Design review of the part built by this model. Coordinates are the model's own, in mm. Round coordinates to 2 decimals unless told otherwise and drop trailing zeros. Loops run counter-clockwise (first coordinate to the right, second up) from the corner with the lowest first, then second, coordinate; pieces in that order, holes last. Notation, with made-up numbers: M 79.25,12.25 L 94.25,12.25 A26 cw 94.25,51.25 Z; hole C 0,42 d8. An arc over 180 degrees is marked long. One line per item, written item: value. Start each with the question number.
Item 1: For line 1 along Z through (x, y) = (-5.5, 31.5); line 2 along Y through (x, z) = (1.75, 0); line 3 along Z through (x, y) = (5.5, -10.5), list the stretches that pass through material, from the lowest coordinate up.
Item 2: Clearance check with flat-ended pins moving along their axes: pin 1 (1.5 mm diameter, centred on x = -5, z = -13, fed in from -Y); pin 2 (6 mm diameter, centred on x = -0.5, y = 47.5, fed in from +Z); pin 3 (8 mm diameter, centred on x = -0.5, z = -27.5, fed in from +Y); pin 4 (6 mm diameter, centred on x = -4, z = -5.5, fed in from +Y). State where each tip first meets the part, or that it passes through.
Item 3: We need section C-C (z = 2.5). Write out the cut boundary in (x, y).
Item 4: We need section A-A (x = -3.25). Write out the cut boundary in (y, z), then the cut area to 3 significant figures.
Item 5: We need section B-B (y = -5). Write out the cut boundary in (x, z).
from build123d import *

# Parameters (mm, degrees)
BOSS_EXTRU_1_DEPTH      = 10
BOSS_EXTRU_1_DEPTH_BACK = 10
ESQUISSE1_R             = 1


with BuildPart() as part:
    # Esquisse1 → Boss.-Extru.1 (new, two sides: drawn at the far end of the back side and taken through both)
    with BuildSketch(Plane(origin=(0, 0, 0), x_dir=(0, 0, -1), z_dir=(1, 0, 0)).offset(-BOSS_EXTRU_1_DEPTH_BACK)):
        Polygon((5.047823589, 2.497154895), (33.133709904, -54.276495693), (23.038062725, -59.270805483), (-5.047823589, -2.497154895), (-5, 60), (5, 60), align=None)
        Circle(ESQUISSE1_R, mode=Mode.SUBTRACT)
    extrude(amount=BOSS_EXTRU_1_DEPTH + BOSS_EXTRU_1_DEPTH_BACK)


solid = part.part
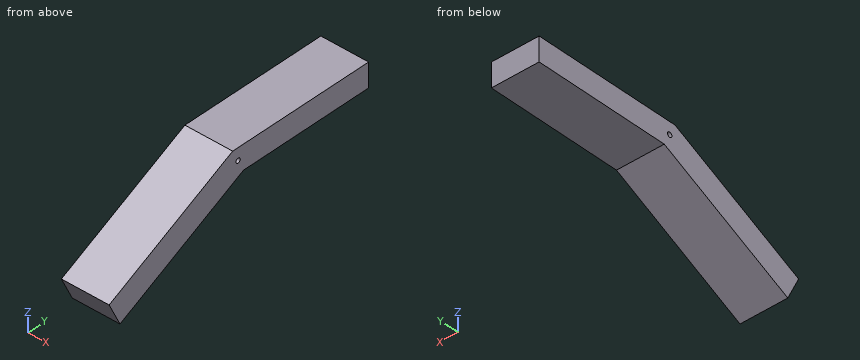
A:
1. line 1: -5.02 to 5.02
1. line 2: -12.7 to -1, 1 to 60
1. line 3: -11.48 to 1.09
2. pin 1: y = -40.5
2. pin 2: z = 5.01
2. pin 3: y = -34.8
2. pin 4: y = 60
3. outline: M -10,-7.65 L 10,-7.65 L 10,60 L -10,60 Z
4. outline: M -59.27,-23.04 L -54.28,-33.13 L 2.5,-5.05 L 60,-5 L 60,5 L -2.5,5.05 Z; hole C 0,0 d2
4. area: 1,310 mm2
5. outline: M -10,-8.76 L 10,-8.76 L 10,3.81 L -10,3.81 Z
